Autodesk Inventor part; units mm, degrees
ref_plane "YZ Plane" through (0, 0, 0) normal (1, 0, 0) x (0, 1, 0)
ref_plane "XZ Plane" through (0, 0, 0) normal (0, 1, 0) x (-1, 0, 0)
ref_plane "XY Plane" through (0, 0, 0) normal (0, 0, 1) x (1, 0, 0)
sketch "Sketch1" plane through (0, 0, 0) normal (0, 0, 1) x (1, 0, 0)
  line L0 (-59.7338, 79.3295) -> (-59.7338, -22.2705)
  line L1 (-59.7338, -22.2705) -> (67.2662, -22.2705)
  line L2 (67.2662, -22.2705) -> (67.2662, 60.2795)
  line L3 (67.2662, 60.2795) -> (19.6412, 60.2795)
  line L4 (19.6412, 60.2795) -> (19.6412, 9.4795)
  line L5 (19.6412, 9.4795) -> (-15.2838, 9.4795)
  line L6 (-15.2838, 9.4795) -> (-15.2838, 79.3295)
  line L7 (-15.2838, 79.3295) -> (-59.7338, 79.3295)
  point P0 (0, 0)
  point P1 (-47.0338, 66.6295)
  point P2 (54.5662, 47.5795)
  point P3 (41.8662, -3.2205)
  point P4 (-47.0338, -9.5705)
  dimension "d0" = 101.6
  dimension "d1" = 127
  dimension "d2" = 44.45
  dimension "d3" = 47.625
  dimension "d4" = 82.55
  dimension "d5" = 69.85
  dimension "d6" = 12.7
  dimension "d7" = 12.7
  dimension "d8" = 12.7
  dimension "d9" = 12.7
  dimension "d10" = 19.05
  dimension "d11" = 25.4
  dimension "d21" = 12.7
  dimension "d22" = 12.7
extrude "Extrusion1" add sketch "Sketch1" against normal blind 3.175
hole "Hole1" at (-47.0338, 66.6295, 0) at (54.5662, 47.5795, 0) at (41.8662, -3.2205, 0) direction (0, 0, -1) diameter 6.35 depth 25.4 tip angle 118
hole "Hole2" at (-47.0338, -9.5705, 0) direction (0, 0, -1) diameter 6.35 end through all
properties part number "AS5-8-4-001"
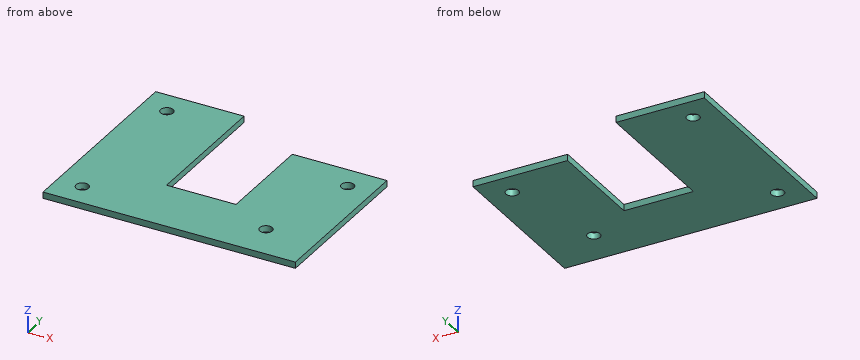
Read the model definition and answer for the solid it produces. Units are mm, in the model's axes. Round coordinates to 2 decimals unless told otherwise and drop trailing zeros. Write each loop counter-clockwise with the first axis right and the second up, starting at its lowest first coordinate (ties: lowest second). Pieces come first, ordered by that corner, then holes. Notation, with made-up numbers: (47, 55.25) - (78, 55.25) arc R28 ccw to (78, 75.25) - close; hole circle Ø1 at (-30.75, 39.25). An arc over 180 degrees is marked (long way). Use a Markdown table: item, result.
(1) The part is cut by section C-C (y = 47.5). Write down the section's boundary in (x, z) (3 decimals), then the cut area to 3 significant figures.
Reported:
| item | result |
|---|---|
| outline | (-59.734, -3.175) - (-15.284, -3.175) - (-15.284, 0) - (-59.734, 0) - close; (19.641, -3.175) - (51.392, -3.175) - (51.392, 0) - (19.641, 0) - close; (57.74, -3.175) - (67.266, -3.175) - (67.266, 0) - (57.74, 0) - close |
| area | 272 mm2 |
(2) Straight lines are drawn through the part: line 1 along X through (y, z) = (18, -2.15); line 2 along Y through (x, z) = (-47, -2.7); line 3 along Y through (x, z) = (-45.5, -1.5). For each, find the intervals that lie inside material, in ascending order. Write a range as [from, to].
Reported:
| item | result |
|---|---|
| line 1 | [-59.73, -15.28], [19.64, 67.27] |
| line 2 | [-22.27, -12.75], [-6.4, 63.45], [69.8, 79.33] |
| line 3 | [-22.27, -12.35], [-6.79, 63.85], [69.41, 79.33] |
(3) The part is cut by section A-A (y = 19). Write down the section's boundary in (x, z) (3 decimals).
Reported:
| item | result |
|---|---|
| outline | (-59.734, -3.175) - (-15.284, -3.175) - (-15.284, 0) - (-59.734, 0) - close; (19.641, -3.175) - (67.266, -3.175) - (67.266, 0) - (19.641, 0) - close |
(4) The part is cut by section B-B (z = -1.3). State how many separate pieces and enclosed holes the cut face has, then the cut area to 3 significant figures.
Reported:
| item | result |
|---|---|
| separate pieces | 1 |
| enclosed holes | 4 |
| area | 9,430 mm2 |
(5) The part is cut by section D-D (x = 7). Write down the section's boundary in (y, z) (1 decimal), then the cut area to 3 significant figures.
Reported:
| item | result |
|---|---|
| outline | (-22.3, -3.2) - (9.5, -3.2) - (9.5, 0) - (-22.3, 0) - close |
| area | 101 mm2 |
(6) Each of these flat-tipped pins is pushed along its axis until it touches: pin 1 Ø1 at (x, z) = (4.5, -2) entering from +Y; pin 2 Ø4 at (x, y) = (41.87, -3.22) entering from -Z. Where does it stop, or does it pass through?
Reported:
| item | result |
|---|---|
| pin 1 | y = 9.48 |
| pin 2 | through |
